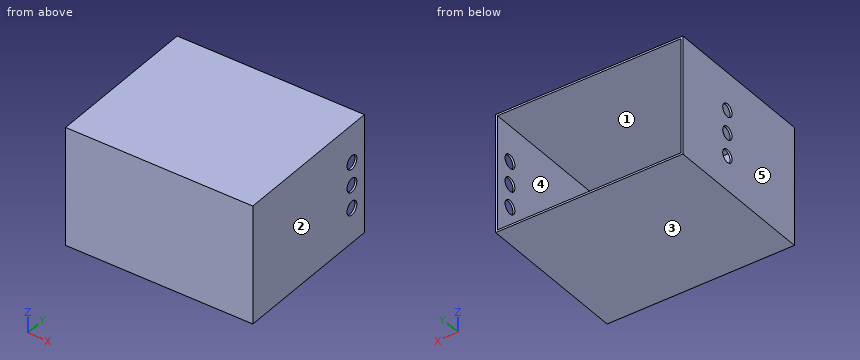
```python
from build123d import *

# Parameters (mm, degrees)
SKETCH1_W                = 152.4
SKETCH1_H                = 190.5
BOSS_EXTRUDE1_DEPTH      = 5.08
BOSS_EXTRUDE2_DEPTH      = 254
BOSS_EXTRUDE2_DEPTH_BACK = 5.08
SKETCH2_W                = 311.15
SKETCH2_H                = 196.85
SKETCH3_W                = 304.8
SKETCH3_H                = 190.5
CUT_EXTRUDE1_DEPTH       = 252.73
SKETCH4_R                = 10.75942509
CUT_EXTRUDE2_DEPTH       = 252.73
SKETCH5_R                = 11.36861001
CUT_EXTRUDE3_DEPTH       = 252.73


with BuildPart() as part:
    # Sketch1 → Boss-Extrude1 (new body)
    with BuildSketch(Plane(origin=(0, 0, 0), x_dir=(1, 0, 0), z_dir=(0, 1, 0))):
        with Locations((-76.2, 0)):
            Rectangle(SKETCH1_W, SKETCH1_H)
    extrude(amount=BOSS_EXTRUDE1_DEPTH)

    # Sketch2 → Boss-Extrude2 (add, two sides: drawn at the far end of the back side and taken through both)
    with BuildSketch(Plane(origin=(0, 5.08, 0), x_dir=(1, 0, 0), z_dir=(0, 1, 0)).offset(-BOSS_EXTRUDE2_DEPTH_BACK)):
        Rectangle(SKETCH2_W, SKETCH2_H)
    extrude(amount=BOSS_EXTRUDE2_DEPTH + BOSS_EXTRUDE2_DEPTH_BACK)

    # Sketch3 → Cut-Extrude1 (cut)
    with BuildSketch(Plane(origin=(0, 259.08, 0), x_dir=(1, 0, 0), z_dir=(0, 1, 0))):
        Rectangle(SKETCH3_W, SKETCH3_H)
    extrude(amount=-CUT_EXTRUDE1_DEPTH, mode=Mode.SUBTRACT)

    # Sketch4 → Cut-Extrude2 (cut)
    with BuildSketch(Plane.ZY.offset(155.575)):
        with Locations((-40.782647245, 155.631127926)):
            Circle(SKETCH4_R)
        with Locations((-2.682647245, 155.631127926)):
            Circle(SKETCH4_R)
        with Locations((35.417352755, 155.631127926)):
            Circle(SKETCH4_R)
    extrude(amount=-CUT_EXTRUDE2_DEPTH, mode=Mode.SUBTRACT)

    # Sketch5 → Cut-Extrude3 (cut)
    with BuildSketch(Plane(origin=(155.575, 0, 0), x_dir=(0, 0, -1), z_dir=(1, 0, 0))):
        with Locations((-35.725024922, 230.210156067)):
            Circle(SKETCH5_R)
        with Locations((2.374975078, 230.210156067)):
            Circle(SKETCH5_R)
        with Locations((40.474975078, 230.210156067)):
            Circle(SKETCH5_R)
    extrude(amount=-CUT_EXTRUDE3_DEPTH, mode=Mode.SUBTRACT)


solid = part.part
```
Could you check a few things on this model? Use its own coordinates, in mm. Face numbers are marked on the shaded views. A direction names the side the tool comes from. Round coordinates to 2 decimals unless told otherwise and drop trailing zeros. Loops run counter-clockwise (first coordinate to the right, second up) from the corner with the lowest first, then second, coordinate; pieces in that order, holes last. Notation, with made-up numbers: (-39, 9.5) -> (-6, 9.5) arc R9 cw to (-6, 26.5) -> close; hole circle Ø3 at (-2.5, -4). An arc over 180 degrees is marked (long way). One line per question, with ' | ' between items.
(1) If we section it at D-D on y = 236: List the corners of the cut face in (x, z) for me (3 decimals).
Model answer:
outline: (-155.575, -98.425) -> (155.575, -98.425) -> (155.575, -50.259) -> (152.4, -50.259) -> (152.4, -95.25) -> (-152.4, -95.25) -> (-152.4, 95.25) -> (152.4, 95.25) -> (152.4, 45.509) -> (155.575, 45.509) -> (155.575, 98.425) -> (-155.575, 98.425) -> close; (152.4, -30.691) -> (155.575, -30.691) -> (155.575, -12.159) -> (152.4, -12.159) -> close; (152.4, 7.409) -> (155.575, 7.409) -> (155.575, 25.941) -> (152.4, 25.941) -> close
(2) If we section it at B-B on z = -19.5: List the corners of the cut face in (x, y) for me (3 decimals), and give its area (3 significant figures).
Model answer:
outline: (-155.575, 0) -> (155.575, 0) -> (155.575, 259.08) -> (152.4, 259.08) -> (152.4, 6.35) -> (-152.4, 6.35) -> (-152.4, 259.08) -> (-155.575, 259.08) -> close | area: 3,580 mm^2
(3) For pin 1 Ø18 at (y, z) = (230.21, 35.73) entering from +X; pin 2 Ø8 at (x, z) = (46, -19) entering from -Y; pin 3 Ø1 at (x, z) = (-106, -38.5) entering from +Y, each with a flat end and sliding along its axis, tell me the tip position at first contact or that it passes through.
Model answer:
pin 1: stops at x = -152.4 | pin 2: stops at y = 0 | pin 3: stops at y = 6.35
(4) For the marked faces 1 and 2, which set-ups out of +Z, -Z, +X, -X, +Y, -Y let a thin tool reach every point of the face, with its end or its side?
Model answer:
face 1: +Y | face 2: +Z, -Z, +X, +Y, -Y
(5) If I drill on probe 1 along X at (y, z) = (244, -59) (3 decimals); probe 2 along Z at (x, y) = (59.5, 77) (3 decimals); probe 3 along Y at (x, z) = (-40.5, -6.5), over which ranges is the centre line in solid material (lowest first)?
Model answer:
probe 1: x = -155.575 to -152.4, 152.4 to 155.575 | probe 2: z = -98.425 to -95.25, 95.25 to 98.425 | probe 3: y = 0 to 6.35
(6) If we section it at C-C on x = 125.5: List the corners of the cut face in (y, z) for me (3 decimals).
Model answer:
outline: (0, -98.425) -> (259.08, -98.425) -> (259.08, -95.25) -> (6.35, -95.25) -> (6.35, 95.25) -> (259.08, 95.25) -> (259.08, 98.425) -> (0, 98.425) -> close
(7) Thinking about a two-plate mould opening in Z: for the marked faces 3, 4 and 5, which applies, released by +Z, released by -Z, zero draft, split by the parting line, or undercut?
Model answer:
face 3: released by -Z | face 4: undercut | face 5: zero draft
(8) If we section it at A-A on y = 99.5: List the corners of the cut face in (x, z) for me (3 decimals), and give its area (3 significant figures).
Model answer:
outline: (-155.575, -98.425) -> (155.575, -98.425) -> (155.575, 98.425) -> (-155.575, 98.425) -> close; hole (-152.4, -95.25) -> (152.4, -95.25) -> (152.4, 95.25) -> (-152.4, 95.25) -> close | area: 3,190 mm^2
